```python
from build123d import *

# Parameters (mm, degrees)
SKETCH1_W           = 21
SKETCH1_H           = 64.5
BOSS_EXTRUDE1_DEPTH = 18.7
CUT_EXTRUDE1_DEPTH  = 22
SKETCH3_W           = 3.2
SKETCH3_H           = 4.5
CUT_EXTRUDE2_DEPTH  = 3


with BuildPart() as part:
    # Sketch1 → Boss-Extrude1 (new body)
    with BuildSketch(Plane(origin=(0, 0, 0), x_dir=(1, 0, 0), z_dir=(0, 1, 0))):
        with Locations((-10.5, -32.25)):
            Rectangle(SKETCH1_W, SKETCH1_H)
    extrude(amount=BOSS_EXTRUDE1_DEPTH)

    # Sketch2 → Cut-Extrude1 (cut, through all)
    with BuildSketch(Plane(origin=(0, 0, 0), x_dir=(0, 0, -1), z_dir=(1, 0, 0))):
        Polygon((-59.5, 0), (-5, 0), (-5, 4.5), (-26.5, 4.5), (-26.5, 16.7), (-49.5, 16.7), (-49.5, 4.5), (-59.5, 4.5), align=None)
    extrude(amount=-CUT_EXTRUDE1_DEPTH, mode=Mode.SUBTRACT)

    # Sketch3 → Cut-Extrude2 (cut)
    with BuildSketch(Plane(origin=(0, 0, 59.5), x_dir=(-1, 0, 0), z_dir=(0, 0, -1))):
        with Locations((13.9, 2.25)):
            Rectangle(SKETCH3_W, SKETCH3_H)
    extrude(amount=-CUT_EXTRUDE2_DEPTH, mode=Mode.SUBTRACT)


solid = part.part
```
Design review of the part built by this model. Coordinates are the model's own, in mm. A direction names the side the tool comes from. Round coordinates to 2 decimals unless told otherwise and drop trailing zeros. Write each loop counter-clockwise with the first axis right and the second up, starting at its lowest first coordinate (ties: lowest second). Pieces come first, ordered by that corner, then holes. Notation, with made-up numbers: (19.5, 20) -> (70.5, 20) arc R20 cw to (70.5, 44) -> close; hole circle Ø8 at (-23, 13). An arc over 180 degrees is marked (long way). Answer in a Markdown table with one row per item.
Q1. For faces 1 (the face through (-14, 2, 62.5)), 2 (the face through (-10, 11, 26.5)), 3 (the face through (-11, 0, 62)), list the 3-axis set-ups (+Z, -Z, +X, -X, +Y, -Y) from which the entire face can be reached by the end or side of a thin tool; tool diameter is ignored.
The answers:
| item | result |
|---|---|
| face 1 | -Y |
| face 2 | +X, -X, -Y |
| face 3 | +Z, -Z, +X, -X, -Y |
Q2. Draft analysis for pull direction X (two halves, no side actions). For faces 4 (the face through (-12.3, 2, 61)), 5 (the face through (-11, 0, 2)), 6 (the face through (0, 11, 26)), 7 (the face through (-15.5, 2, 61)), state which applies: +X half, -X half, draft (parallel to the pull), parting line (faces both ways), or undercut.
The answers:
| item | result |
|---|---|
| face 4 | undercut |
| face 5 | draft |
| face 6 | +X half |
| face 7 | undercut |
Q3. Clearance check with flat-ended pins moving along their axes: pin 1 Ø12 at (x, z) = (-14.5, 34.5) entering from -Y; pin 2 Ø4 at (x, z) = (-18, 19.5) entering from -Y. State where each tip first meets the part, or that it passes through.
The answers:
| item | result |
|---|---|
| pin 1 | y = 16.7 |
| pin 2 | y = 4.5 |
Q4. Take a section at D-D, the plane z = 41. State the section outline as (x, y) points.
The answers:
| item | result |
|---|---|
| outline | (-21, 16.7) -> (0, 16.7) -> (0, 18.7) -> (-21, 18.7) -> close |
Q5. Take a section at B-B, the plane x = -8.5. State the section outline as (y, z) points.
The answers:
| item | result |
|---|---|
| outline | (0, 0) -> (18.7, 0) -> (18.7, 64.5) -> (0, 64.5) -> (0, 59.5) -> (4.5, 59.5) -> (4.5, 49.5) -> (16.7, 49.5) -> (16.7, 26.5) -> (4.5, 26.5) -> (4.5, 5) -> (0, 5) -> close |
Q6. Take a section at A-A, the plane y = 10.5. State the section outline as (x, z) points, then the cut area to 4 significant figures.
The answers:
| item | result |
|---|---|
| outline | (-21, 0) -> (0, 0) -> (0, 26.5) -> (-21, 26.5) -> close; (-21, 49.5) -> (0, 49.5) -> (0, 64.5) -> (-21, 64.5) -> close |
| area | 871.5 mm² |
Q7. To check wall thickness, follow L1, parallel to Z at x = -16, y = 6.25; L2, parallel to Y at x = -17, z = 25; L3, parallel to Y at x = -17, z = 47.5. State the ranges of each line that lie inside material, in increasing order. Write a range as [from, to].
The answers:
| item | result |
|---|---|
| L1 | [0, 26.5], [49.5, 64.5] |
| L2 | [4.5, 18.7] |
| L3 | [16.7, 18.7] |
Q8. Take a section at C-C, the plane y = 3. State the section outline as (x, z) points.
The answers:
| item | result |
|---|---|
| outline | (-21, 0) -> (0, 0) -> (0, 5) -> (-21, 5) -> close; (-21, 59.5) -> (-15.5, 59.5) -> (-15.5, 62.5) -> (-12.3, 62.5) -> (-12.3, 59.5) -> (0, 59.5) -> (0, 64.5) -> (-21, 64.5) -> close |
